```python
from build123d import *

# Parameters (mm, degrees)
SKETCH1_W           = 38.1
SKETCH1_H           = 63.5
SKETCH1_W_2         = 31.75
SKETCH1_H_2         = 57.15
BOSS_EXTRUDE1_DEPTH = 635
CUT_EXTRUDE1_REACH  = 638.934
SKETCH2_R           = 19.05


with BuildPart() as part:
    # Sketch1 → Boss-Extrude1 (new body)
    with BuildSketch(Plane.XY):
        Rectangle(SKETCH1_W, SKETCH1_H)
        Rectangle(SKETCH1_W_2, SKETCH1_H_2, mode=Mode.SUBTRACT)
    extrude(amount=BOSS_EXTRUDE1_DEPTH)

    # Cut-Extrude1: up to this face of the body (flat: up to its plane)
    cut_extrude1_end = Plane(part.part.faces().sort_by_distance((-19.05, 0, 317.5))[0])
    # Sketch2 → Cut-Extrude1 (cut, up to the picked face)
    with BuildSketch(Plane(origin=(19.05, 0, 0), x_dir=(0, 0, -1), z_dir=(1, 0, 0)), mode=Mode.PRIVATE) as cut_extrude1_sk1:
        with Locations((-560.5018, 0)):
            Circle(SKETCH2_R)
    cut_extrude1_tool1 = split(extrude(cut_extrude1_sk1.sketch, amount=-CUT_EXTRUDE1_REACH, mode=Mode.PRIVATE), bisect_by=cut_extrude1_end, keep=Keep.BOTH, mode=Mode.PRIVATE)
    # Sketch2 → Cut-Extrude1 (cut, up to the picked face)
    with BuildSketch(Plane(origin=(19.05, 0, 0), x_dir=(0, 0, -1), z_dir=(1, 0, 0)), mode=Mode.PRIVATE) as cut_extrude1_sk2:
        with Locations((-497.0018, 0)):
            Circle(SKETCH2_R)
    cut_extrude1_tool2 = split(extrude(cut_extrude1_sk2.sketch, amount=-CUT_EXTRUDE1_REACH, mode=Mode.PRIVATE), bisect_by=cut_extrude1_end, keep=Keep.BOTH, mode=Mode.PRIVATE)
    # Sketch2 → Cut-Extrude1 (cut, up to the picked face)
    with BuildSketch(Plane(origin=(19.05, 0, 0), x_dir=(0, 0, -1), z_dir=(1, 0, 0)), mode=Mode.PRIVATE) as cut_extrude1_sk3:
        with Locations((-433.5018, 0)):
            Circle(SKETCH2_R)
    cut_extrude1_tool3 = split(extrude(cut_extrude1_sk3.sketch, amount=-CUT_EXTRUDE1_REACH, mode=Mode.PRIVATE), bisect_by=cut_extrude1_end, keep=Keep.BOTH, mode=Mode.PRIVATE)
    # Sketch2 → Cut-Extrude1 (cut, up to the picked face)
    with BuildSketch(Plane(origin=(19.05, 0, 0), x_dir=(0, 0, -1), z_dir=(1, 0, 0)), mode=Mode.PRIVATE) as cut_extrude1_sk4:
        with Locations((-370.0018, 0)):
            Circle(SKETCH2_R)
    cut_extrude1_tool4 = split(extrude(cut_extrude1_sk4.sketch, amount=-CUT_EXTRUDE1_REACH, mode=Mode.PRIVATE), bisect_by=cut_extrude1_end, keep=Keep.BOTH, mode=Mode.PRIVATE)
    # Sketch2 → Cut-Extrude1 (cut, up to the picked face)
    with BuildSketch(Plane(origin=(19.05, 0, 0), x_dir=(0, 0, -1), z_dir=(1, 0, 0)), mode=Mode.PRIVATE) as cut_extrude1_sk5:
        with Locations((-306.5018, 0)):
            Circle(SKETCH2_R)
    cut_extrude1_tool5 = split(extrude(cut_extrude1_sk5.sketch, amount=-CUT_EXTRUDE1_REACH, mode=Mode.PRIVATE), bisect_by=cut_extrude1_end, keep=Keep.BOTH, mode=Mode.PRIVATE)
    # Sketch2 → Cut-Extrude1 (cut, up to the picked face)
    with BuildSketch(Plane(origin=(19.05, 0, 0), x_dir=(0, 0, -1), z_dir=(1, 0, 0)), mode=Mode.PRIVATE) as cut_extrude1_sk6:
        with Locations((-243.0018, 0)):
            Circle(SKETCH2_R)
    cut_extrude1_tool6 = split(extrude(cut_extrude1_sk6.sketch, amount=-CUT_EXTRUDE1_REACH, mode=Mode.PRIVATE), bisect_by=cut_extrude1_end, keep=Keep.BOTH, mode=Mode.PRIVATE)
    # Sketch2 → Cut-Extrude1 (cut, up to the picked face)
    with BuildSketch(Plane(origin=(19.05, 0, 0), x_dir=(0, 0, -1), z_dir=(1, 0, 0)), mode=Mode.PRIVATE) as cut_extrude1_sk7:
        with Locations((-179.5018, 0)):
            Circle(SKETCH2_R)
    cut_extrude1_tool7 = split(extrude(cut_extrude1_sk7.sketch, amount=-CUT_EXTRUDE1_REACH, mode=Mode.PRIVATE), bisect_by=cut_extrude1_end, keep=Keep.BOTH, mode=Mode.PRIVATE)
    # Sketch2 → Cut-Extrude1 (cut, up to the picked face)
    with BuildSketch(Plane(origin=(19.05, 0, 0), x_dir=(0, 0, -1), z_dir=(1, 0, 0)), mode=Mode.PRIVATE) as cut_extrude1_sk8:
        with Locations((-116.0018, 0)):
            Circle(SKETCH2_R)
    cut_extrude1_tool8 = split(extrude(cut_extrude1_sk8.sketch, amount=-CUT_EXTRUDE1_REACH, mode=Mode.PRIVATE), bisect_by=cut_extrude1_end, keep=Keep.BOTH, mode=Mode.PRIVATE)
    # Sketch2 → Cut-Extrude1 (cut, up to the picked face)
    with BuildSketch(Plane(origin=(19.05, 0, 0), x_dir=(0, 0, -1), z_dir=(1, 0, 0)), mode=Mode.PRIVATE) as cut_extrude1_sk9:
        with Locations((-52.5018, 0)):
            Circle(SKETCH2_R)
    cut_extrude1_tool9 = split(extrude(cut_extrude1_sk9.sketch, amount=-CUT_EXTRUDE1_REACH, mode=Mode.PRIVATE), bisect_by=cut_extrude1_end, keep=Keep.BOTH, mode=Mode.PRIVATE)
    add(cut_extrude1_tool1.solids().sort_by(Axis((19.05, 0, 560.5018), (-1, 0, 0)))[0], mode=Mode.SUBTRACT)
    add(cut_extrude1_tool2.solids().sort_by(Axis((19.05, 0, 497.0018), (-1, 0, 0)))[0], mode=Mode.SUBTRACT)
    add(cut_extrude1_tool3.solids().sort_by(Axis((19.05, 0, 433.5018), (-1, 0, 0)))[0], mode=Mode.SUBTRACT)
    add(cut_extrude1_tool4.solids().sort_by(Axis((19.05, 0, 370.0018), (-1, 0, 0)))[0], mode=Mode.SUBTRACT)
    add(cut_extrude1_tool5.solids().sort_by(Axis((19.05, 0, 306.5018), (-1, 0, 0)))[0], mode=Mode.SUBTRACT)
    add(cut_extrude1_tool6.solids().sort_by(Axis((19.05, 0, 243.0018), (-1, 0, 0)))[0], mode=Mode.SUBTRACT)
    add(cut_extrude1_tool7.solids().sort_by(Axis((19.05, 0, 179.5018), (-1, 0, 0)))[0], mode=Mode.SUBTRACT)
    add(cut_extrude1_tool8.solids().sort_by(Axis((19.05, 0, 116.0018), (-1, 0, 0)))[0], mode=Mode.SUBTRACT)
    add(cut_extrude1_tool9.solids().sort_by(Axis((19.05, 0, 52.5018), (-1, 0, 0)))[0], mode=Mode.SUBTRACT)


solid = part.part
```
Check sheet for the modelled part. Datum: model origin and axes. Units: mm. A direction names the side the tool comes from. Give positions to 0.01 mm unless a question says otherwise; leave off trailing zeros. Write each loop counter-clockwise with the first axis right and the second up, starting at its lowest first coordinate (ties: lowest second). Pieces come first, ordered by that corner, then holes.
Item 1: Gauge pin test, flat end, axial feed: pin 1 (8 mm diameter, centred on y = -5, z = 357, fed in from +X). Record the tip position at first contact, or that the pin passes through.
Item 2: Cross-section at C-C (y = 0). Count the separate pieces of the cut face and the enclosed holes in it, and give its area (3 significant figures).
Item 3: Cross-section at B-B (z = 463.5). Enter the section's corners in (x, y) (3 decimals).
Item 4: Access from +Z, -Z, +X, -X, +Y, -Y to the whole of each face (thin tool, end or side, straight path). Record for faces 1 (the face through (0, 28.575, 313)), 2 (the face through (-17.44, -18.597, 56.631)).
Item 5: Cross-section at A-A (x = -8.5). Enter the section's corners in (y, z) (3 decimals).
Item 6: Draft check along Y on faces 3 (the face through (-17, 3, 635)), 4 (the face through (-17.44, 5.72, 97.83)), 5 (the face through (0, 31.75, 313)), 6 (the face through (-17.44, 0.838, 452.533)). Enter one of: released by +Y, released by -Y, zero draft, split by the parting line, or undercut.
Item 7: Scan lines: L1, parallel to Y at x = 6.5, z = 42 (3 decimals); L2, parallel to X at y = 7, z = 461.5 (3 decimals). Record each from-to range of solid material in increasing order.
Report:
1. pin 1: passes through
2. separate pieces: 20
2. enclosed holes: 0
2. area: 1,850 mm2
3. outline: (-19.05, -31.75) - (19.05, -31.75) - (19.05, 31.75) - (-19.05, 31.75) - close; hole (-15.875, -28.575) - (15.875, -28.575) - (15.875, 28.575) - (-15.875, 28.575) - close
4. face 1: +Z, -Z
4. face 2: +X, -X
5. outline: (-31.75, 0) - (-28.575, 0) - (-28.575, 635) - (-31.75, 635) - close; (28.575, 0) - (31.75, 0) - (31.75, 635) - (28.575, 635) - close
6. face 3: zero draft
6. face 4: undercut
6. face 5: released by +Y
6. face 6: undercut
7. L1: y = -31.75 to -28.575, 28.575 to 31.75
7. L2: x = -19.05 to -15.875, 15.875 to 19.05
